Source: CAD feature listing. Evaluate the final solid. Frame: model axes, mm. A direction names the side the tool comes from. Coordinates: 2 decimals unless noted, no trailing zeros. Loops run counter-clockwise (first coordinate to the right, second up) from the corner with the lowest first, then second, coordinate; pieces in that order, holes last. Notation, with made-up numbers: (78, -37.75) -> (119, -37.75) arc R9 ccw to (119, -25.75) -> close; hole circle Ø3 at (17.5, 40.25). An arc over 180 degrees is marked (long way). Answer as a JSON object with one key per item and string values. Group by question number.
from build123d import *

# Parameters (mm, degrees)
EXTRUDE_2_DEPTH     = 6
SKETCH_2_R          = 1.55
CUT_EXTRUDE_1_DEPTH = 10
SKETCH_3_R          = 1.55
CUT_EXTRUDE_2_DEPTH = 10
SKETCH_5_R          = 2.5
EXTRUDE_3_DEPTH     = 50


with BuildPart() as part:
    # 草图1 → 凸台-拉伸2 (new body)
    with BuildSketch(Plane(origin=(0, 0, 0), x_dir=(1, 0, 0), z_dir=(0, 1, 0))):
        Polygon((-72.757575758, -68.484848485), (-72.757575758, -1.484848485), (71.242424242, -1.484848485), (71.242424242, -68.484848485), (74.242424242, -68.484848485), (74.242424242, -1.484848485), (74.242424242, 1.515151515), (71.242424242, 1.515151515), (-72.757575758, 1.515151515), (-75.757575758, 1.515151515), (-75.757575758, -1.484848485), (-75.757575758, -68.484848485), align=None)
    extrude(amount=EXTRUDE_2_DEPTH)

    # 草图2 → 切除-拉伸1 (cut)
    with BuildSketch(Plane(origin=(-72.757575758, 0, 0), x_dir=(0, 0, -1), z_dir=(1, 0, 0))):
        with Locations((-65.484848485, 3)):
            Circle(SKETCH_2_R)
    extrude(amount=-CUT_EXTRUDE_1_DEPTH, mode=Mode.SUBTRACT)

    # 草图3 → 切除-拉伸2 (cut)
    with BuildSketch(Plane(origin=(74.242424242, 0, 0), x_dir=(0, 0, -1), z_dir=(1, 0, 0))):
        with Locations((-65.484848485, 3)):
            Circle(SKETCH_3_R)
    extrude(amount=-CUT_EXTRUDE_2_DEPTH, mode=Mode.SUBTRACT)

    # 草图5 → 凸台-拉伸3 (add)
    with BuildSketch(Plane(origin=(0, 0, -1.515151515), x_dir=(-1, 0, 0), z_dir=(0, 0, -1))):
        with Locations(Location((0.757575758, 3, 0), (0, 0, 180))):
            Circle(SKETCH_5_R)
    extrude(amount=EXTRUDE_3_DEPTH)


solid = part.part
1. Reachability of faces 1 (the face through (-2.74, 4.52, -26.17)), 2 (the face through (-34, 0, 0)), 3 (the face through (-2, 3, 1.485)) from +Z, -Z, +X, -X, +Y, -Y: full face, straight path, thin tool, end or side. Return the list, or none.
2. Section query A-A on y = 3. Return loops of the section in (x, z), then the cut area to 3 significant figures.
3. Section query D-D on z = -8.5. Return loops of the section in (x, y), then the cut area to 3 significant figures.
4. Section query C-C on x = -24. Return loops of the section in (y, z), then the cut area to 3 significant figures.
5. Section query B-B on z = 43. Return loops of the section in (x, y).
6. Mould query, pull axis Z, two halves, no side actions, for faces 4 (the face through (0.3, 0.3, -1.515)), 5 (the face through (71.242, 3, 35)), 6 (the face through (72.763, 3.466, 64.006)). Classes: pulls with the +Z half, pulls with the -Z half, needs draft (parallel to the pull), parting line crosses it, or undercut.
7. Ray query, L1, parallel to X at y = 0.4, z = 21.5; L2, parallel to Z at x = 51.5, y = 5.25; L3, parallel to X at y = 5.2, z = -41 (3 decimals). Return the intervals inside material, ascending.
8. Pin query (flat end, axial travel): pin 1 Ø1.9 at (y, z) = (3, 65.48) entering from +X; pin 2 Ø1.8 at (x, y) = (19.5, 4) entering from -Z; pin 3 Ø1 at (x, y) = (-24.5, 1) entering from +Z. Return the tip coordinate at first contact, or that it passes through.
Solved:
{
 "1": {"face 1": "-Z", "face 2": "+Z, -Z, +X, -X, -Y", "face 3": "+Z, +Y, -Y"},
 "2": {"outline": "(-75.76, -1.52) -> (-3.26, -1.52) -> (-3.26, -51.52) -> (1.74, -51.52) -> (1.74, -1.52) -> (74.24, -1.52) -> (74.24, 63.93) -> (71.24, 63.93) -> (71.24, 1.48) -> (-72.76, 1.48) -> (-72.76, 63.93) -> (-75.76, 63.93) -> close; (-75.76, 67.03) -> (-72.76, 67.03) -> (-72.76, 68.48) -> (-75.76, 68.48) -> close; (71.24, 67.03) -> (74.24, 67.03) -> (74.24, 68.48) -> (71.24, 68.48) -> close", "area": "1,080 mm^2"},
 "3": {"outline": "circle Ø5 at (-0.76, 3)", "area": "19.6 mm^2"},
 "4": {"outline": "(0, -1.52) -> (6, -1.52) -> (6, 1.48) -> (0, 1.48) -> close", "area": "18.0 mm^2"},
 "5": {"outline": "(-75.76, 0) -> (-72.76, 0) -> (-72.76, 6) -> (-75.76, 6) -> close; (71.24, 0) -> (74.24, 0) -> (74.24, 6) -> (71.24, 6) -> close"},
 "6": {"face 4": "pulls with the -Z half", "face 5": "needs draft", "face 6": "undercut"},
 "7": {"L1": "-75.76 to -72.76, 71.24 to 74.24", "L2": "-1.52 to 1.48", "L3": "-1.945 to 0.43"},
 "8": {"pin 1": "through", "pin 2": "z = -1.52", "pin 3": "z = 1.48"}
}
